Autodesk Inventor part; units mm, degrees
ref_plane "YZ Plane" through (0, 0, 0) normal (1, 0, 0) x (0, 1, 0)
ref_plane "XZ Plane" through (0, 0, 0) normal (0, 1, 0) x (-1, 0, 0)
ref_plane "XY Plane" through (0, 0, 0) normal (0, 0, 1) x (1, 0, 0)
sketch "Sketch1" plane through (0, 0, 0) normal (0, 1, 0) x (-1, 0, 0)
  circle A0 centre (0, 0) radius 12.5
  circle A1 centre (0, 0) radius 22.5
  line L0 (12.5, 0) -> (22.5, 0)
  line L1 (12.2268, 2.5989) -> (22.0083, 4.678)
  line L2 (11.4193, 5.0842) -> (20.5548, 9.1516)
  line L3 (10.1127, 7.3473) -> (18.2029, 13.2252)
  line L4 (8.3641, 9.2893) -> (15.0554, 16.7208)
  line L5 (6.25, 10.8253) -> (11.25, 19.4856)
  line L6 (3.8627, 11.8882) -> (6.9529, 21.3988)
  line L7 (1.3066, 12.4315) -> (2.3519, 22.3767)
  line L8 (-1.3066, 12.4315) -> (-2.3519, 22.3767)
  line L9 (-3.8627, 11.8882) -> (-6.9529, 21.3988)
  line L10 (-6.25, 10.8253) -> (-11.25, 19.4856)
  line L11 (-8.3641, 9.2893) -> (-15.0554, 16.7208)
  line L12 (-10.1127, 7.3473) -> (-18.2029, 13.2252)
  line L13 (-11.4193, 5.0842) -> (-20.5548, 9.1516)
  line L14 (-12.2268, 2.5989) -> (-22.0083, 4.678)
  line L15 (-12.5, 0) -> (-22.5, 0)
  line L16 (-12.2268, -2.5989) -> (-22.0083, -4.678)
  line L17 (-11.4193, -5.0842) -> (-20.5548, -9.1516)
  line L18 (-10.1127, -7.3473) -> (-18.2029, -13.2252)
  line L19 (-8.3641, -9.2893) -> (-15.0554, -16.7208)
  line L20 (-6.25, -10.8253) -> (-11.25, -19.4856)
  line L21 (-3.8627, -11.8882) -> (-6.9529, -21.3988)
  line L22 (-1.3066, -12.4315) -> (-2.3519, -22.3767)
  line L23 (1.3066, -12.4315) -> (2.3519, -22.3767)
  line L24 (3.8627, -11.8882) -> (6.9529, -21.3988)
  line L25 (6.25, -10.8253) -> (11.25, -19.4856)
  line L26 (8.3641, -9.2893) -> (15.0554, -16.7208)
  line L27 (10.1127, -7.3473) -> (18.2029, -13.2252)
  line L28 (11.4193, -5.0842) -> (20.5548, -9.1516)
  line L29 (12.2268, -2.5989) -> (22.0083, -4.678)
  circle A2 centre (0, 0) radius 4.25
  circle A3 centre (0, 0) radius 20.5
  point P0 (18.7277, 8.3381)
  point P1 (20.052, 4.2622)
  point P2 (20.5, 0)
  point P3 (20.052, -4.2622)
  point P4 (18.7277, -8.3381)
  point P5 (16.5848, -12.0496)
  point P6 (13.7172, -15.2345)
  point P7 (10.25, -17.7535)
  point P8 (6.3348, -19.4967)
  point P9 (2.1428, -20.3877)
  point P10 (-2.1428, -20.3877)
  point P11 (-6.3348, -19.4967)
  point P12 (-10.25, -17.7535)
  point P13 (-13.7172, -15.2345)
  point P14 (-16.5848, -12.0496)
  point P15 (-18.7277, -8.3381)
  point P16 (-20.052, -4.2622)
  point P17 (-20.5, 0)
  point P18 (-20.052, 4.2622)
  point P19 (-18.7277, 8.3381)
  point P20 (-16.5848, 12.0496)
  point P21 (-13.7172, 15.2345)
  point P22 (-10.25, 17.7535)
  point P23 (-6.3348, 19.4967)
  point P24 (-2.1428, 20.3877)
  point P25 (2.1428, 20.3877)
  point P26 (6.3348, 19.4967)
  point P27 (10.25, 17.7535)
  point P28 (13.7172, 15.2345)
  point P29 (16.5848, 12.0496)
  dimension "d0" = 45
  dimension "d1" = 10
  dimension "d17" = 2
  dimension "d6" = 360
  dimension "d11" = 8.5
extrude "Extrusion1" add sketch "Sketch1" along normal blind 2 contours A0 | A0 L1 A3 L0 | L29 A3 L28 A0 | A3 L1 A1 L0 | L0 A1 L29 A3 | A0 L3 A3 L2 | A3 L2 A1 L1 | L29 A1 L28 A3 | A3 L3 A1 L2 | L27 A3 L26 A0 | L28 A1 L27 A3 | A0 L5 A3 L4 | A3 L4 A1 L3 | L27 A1 L26 A3 | A3 L5 A1 L4 | L25 A3 L24 A0 | L26 A1 L25 A3 | A0 L7 A3 L6 | A3 L6 A1 L5 | L25 A1 L24 A3 | A3 L7 A1 L6 | L23 A3 L22 A0 | L24 A1 L23 A3 | A0 L9 A3 L8 | A3 L8 A1 L7 | L23 A1 L22 A3 | A3 L9 A1 L8 | L21 A3 L20 A0 | L22 A1 L21 A3 | A0 L11 A3 L10 | A3 L10 A1 L9 | L21 A1 L20 A3 | A3 L11 A1 L10 | L19 A3 L18 A0 | L20 A1 L19 A3 | A0 L13 A3 L12 | A3 L12 A1 L11 | L19 A1 L18 A3 | A3 L13 A1 L12 | L17 A3 L16 A0 | L18 A1 L17 A3 | A0 L15 A3 L14 | A3 L14 A1 L13 | L17 A1 L16 A3 | A3 L15 A1 L14 | L16 A1 L15 A3
sketch "Sketch3" plane through (0, 2, 0) normal (0, 1, 0) x (1, 0, 0)
  circle A0 centre (0, 0) radius 4.25
  circle A1 centre (0, 0) radius 7.5
  circle A2 centre (0, 0) radius 4.25
  dimension "d19" = 15
extrude "Extrusion3" add sketch "Sketch3" along normal blind 3 and the other way blind 5
chamfer "Chamfer2" distance 3 angle 45 2 edges at (-7.5, 2, 0) (-7.5, 0, 0)
properties part number "rotary encoder"
CAD build for the part. Positions are in the model's coordinates, mm. Coordinates: 2 decimals unless noted, no trailing zeros. Write each loop counter-clockwise with the first axis right and the second up, starting at its lowest first coordinate (ties: lowest second). Pieces come first, ordered by that corner, then holes. Notation, with made-up numbers: M -38.75,60 L -34.75,60 A20 cw -34.75,81 Z; hole C -8.5,16.25 d8. An arc over 180 degrees is marked long. Return JSON: item names as keys, results as strings.
Item 1: Slice it at A-A, the plane x = 0. State how many separate pieces and enclosed holes the cut face has, and give its area (3 significant figures).
Findings below:
{"separate pieces": "3", "enclosed holes": "0", "area": "114 mm2"}
Item 2: Slice it at B-B, the plane z = -14. Write the cut outline in (x, y), and give its area (3 significant figures).
Findings below:
{"outline": "M -17.61,0 L -12.61,0 L -12.61,2 L -17.61,2 Z; M -8.08,0 L -4.55,0 L -4.55,2 L -8.08,2 Z; M -1.47,0 L 1.47,0 L 1.47,2 L -1.47,2 Z; M 4.55,0 L 8.08,0 L 8.08,2 L 4.55,2 Z; M 12.61,0 L 17.61,0 L 17.61,2 L 12.61,2 Z", "area": "40.1 mm2"}
Item 3: Drop flat-ended pins along their axis: pin 1 Ø1 at (x, z) = (13.5, 9) entering from -Y; pin 2 Ø1 at (x, y) = (-17, 1) entering from -Z; pin 3 Ø10 at (x, z) = (0, 0) entering from +Y; pin 4 Ø5 at (x, z) = (-2.5, -13.5) entering from +Y. Give the stop position or say it passes through.
Findings below:
{"pin 1": "stops at y = 0", "pin 2": "stops at z = -15.3", "pin 3": "stops at y = 5", "pin 4": "stops at y = 2"}
Item 4: Slice it at C-C, the plane x = 15.5. Write the cut outline in (y, z), and give its area (3 significant figures).
Findings below:
{"outline": "M 0,-16.31 L 2,-16.31 L 2,-11.26 L 0,-11.26 Z; M 0,-6.9 L 2,-6.9 L 2,-3.29 L 0,-3.29 Z; M 0,0 L 2,0 L 2,3.29 L 0,3.29 Z; M 0,6.9 L 2,6.9 L 2,11.26 L 0,11.26 Z; M 0,13.42 L 2,13.42 L 2,16.31 L 0,16.31 Z", "area": "38.4 mm2"}
Item 5: Probe line 1 (Z direction, x = 16, y = 1.5); line 2 (Z direction, x = -11.5, y = 0.5); line 3 (Z direction, x = 0.5, y = 1.5). List the from-to ranges inside material, lowest first. Write a range as from..to.
Findings below:
{"line 1": "z = -15.82..-11.62, -7.12..-3.4, 0..3.4, 7.12..11.62, 12.82..15.82", "line 2": "z = -19.34..-16.97, -12.77..-8.36, -5.12..4.9, 5.12..8.36, 12.77..19.34", "line 3": "z = -22.49..-4.22, 4.22..12.49, 20.49..22.49"}
Item 6: Slice it at D-D, the plane y = 4.25. Write the cut outline in (x, z).
Findings below:
{"outline": "C 0,0 d16.5; hole C 0,0 d8.5"}
Item 7: Two-plate mould, pull along Z, no slides. Class faces 1 (the flat face through (-5.08, 0.99, -15.64)), 2 (the conical face through (-7.68, 4.81, 0.34)): +Z half, -Z half, draft (parallel to the pull), parting line (faces both ways), or undercut.
Findings below:
{"face 1": "undercut", "face 2": "parting line"}
